from build123d import *

# Parameters (mm, degrees)
F0_W     = 77.7748
F0_H     = 73.4568
F1_DEPTH = 42.291
F3_W     = 38.6588
F3_H     = 36.5252
F4_DEPTH = 64.262
F5_W     = 18.9484
F5_H     = 17.7546
F6_DEPTH = 109.982


with BuildPart() as f1:
    # F0 (on Front) → F1 (new body, symmetric)
    with BuildSketch(Plane.XZ):
        with Locations((-0.265293, -0.804183)):
            Rectangle(F0_W, F0_H)
    extrude(amount=F1_DEPTH, both=True)

    # F3 (on face) → F4 (join)
    with BuildSketch(Plane(origin=(0, 42.291, 0), x_dir=(-1, 0, 0), z_dir=(0, 1, 0))):
        with Locations((-0.297076, -2.281584)):
            Rectangle(F3_W, F3_H)
    extrude(amount=F4_DEPTH)

    # F5 (on face) → F6 (join)
    with BuildSketch(Plane(origin=(0, 106.553, 0), x_dir=(-1, 0, 0), z_dir=(0, 1, 0))):
        with Locations((-0.515443, -2.880927)):
            Rectangle(F5_W, F5_H)
    extrude(amount=F6_DEPTH)


solid = f1.part
The listing builds one solid part. Answer for the finished solid, in the listing's coordinates (mm). A direction names the side the tool comes from. Round coordinates to 2 decimals unless told otherwise and drop trailing zeros. Write each loop counter-clockwise with the first axis right and the second up, starting at its lowest first coordinate (ties: lowest second). Pieces come first, ordered by that corner, then holes. Notation, with made-up numbers: (88.5, 6.5) - (102.5, 6.5) arc R22 cw to (102.5, 20.5) - close; hole circle Ø1 at (25.5, 40). An arc over 180 degrees is marked (long way). Use a Markdown table: item, result. Add a question column.
1. The part is cut by section D-D (z = -3.5). Write down the section's boundary in (x, y) (3 decimals), and give its area (3 significant figures).
2. The part is cut by section A-A (z = 9.5). Write down the section's boundary in (x, y).
3. A tool of negligible diameter and unlimited length cuts with its end or side. For faces 1 (the face through (1, 74, 15.981)), 2 (the face through (-19.032, 74, -3)), 3 (the face through (-1, -1, -37.533)), 4 (the face through (19.626, 74, -3)), 5 (the face through (1, 161, -11.758)), from which of +Z, -Z, +X, -X, +Y, -Y can it reach the whole face along a straight path? Write none if from no direction.
4. The part is cut by section B-B (x = 16). Write down the section's boundary in (y, z), and give its area (3 significant figures).
5. Consider line 1 (Y direction, x = 1, z = 20); line 2 (Y direction, x = -12, z = -0.5); line 3 (Z direction, x = -2.5, y = 78). Determine where each line is inside the solid, lowest interval first.
6. Flat-ended cylindrical pins translate along their axes: P1, Ø11, axis at y = 62, z = -7, coming from the -X side; P2, Ø19.5, axis at x = 0, y = 81.5, coming from the -Z side; P3, Ø5.5, axis at x = 1.5, y = 158, coming from the +Z side; P4, Ø1, axis at y = 152, z = -12.5, coming from the +X side. Find the tip coordinate at first contact, or state that the pin passes through.
7. The part is cut by section C-C (y = 88). Write down the section's boundary in (x, z), and give its area (3 significant figures).
Reported:
| question | item | result |
|---|---|---|
| 1 | outline | (-39.153, -42.291) - (38.622, -42.291) - (38.622, 42.291) - (19.626, 42.291) - (19.626, 106.553) - (9.99, 106.553) - (9.99, 216.535) - (-8.959, 216.535) - (-8.959, 106.553) - (-19.032, 106.553) - (-19.032, 42.291) - (-39.153, 42.291) - close |
| 1 | area | 11,100 mm^2 |
| 2 | outline | (-39.15, -42.29) - (38.62, -42.29) - (38.62, 42.29) - (19.63, 42.29) - (19.63, 106.55) - (-19.03, 106.55) - (-19.03, 42.29) - (-39.15, 42.29) - close |
| 3 | face 1 | +Z, +X, -X, +Y |
| 3 | face 2 | +Z, -Z, -X, +Y |
| 3 | face 3 | -Z, +X, -X, +Y, -Y |
| 3 | face 4 | +Z, -Z, +X, +Y |
| 3 | face 5 | -Z, +X, -X, +Y |
| 4 | outline | (-42.29, -37.53) - (42.29, -37.53) - (42.29, -20.54) - (106.55, -20.54) - (106.55, 15.98) - (42.29, 15.98) - (42.29, 35.92) - (-42.29, 35.92) - close |
| 4 | area | 8,560 mm^2 |
| 5 | line 1 | -42.29 to 42.29 |
| 5 | line 2 | -42.29 to 106.55 |
| 5 | line 3 | -20.54 to 15.98 |
| 6 | P1 | x = -19.03 |
| 6 | P2 | z = -20.54 |
| 6 | P3 | z = 6 |
| 6 | P4 | through |
| 7 | outline | (-19.03, -20.54) - (19.63, -20.54) - (19.63, 15.98) - (-19.03, 15.98) - close |
| 7 | area | 1,410 mm^2 |
